from build123d import *

# Parameters (mm, degrees)
F0_R     = 1.5
F0_R_2   = 5
F1_DEPTH = 2
F2_SCALE = 10


# Not quite as in the source:
# - ends of sketch curves that miss each other by under 0.0002 mm in the source are joined


with BuildPart() as f1:
    # F0 (on Right) → F1 (new body)
    with BuildSketch(Plane.YZ):
        with BuildLine():
            Line((20.303062, 10.815357), (21.213073, 10.271883))
            ThreePointArc((21.213073, 10.271883), (21.5939035848, 10.2168943828), (21.901025054, 10.4486959684))
            Line((21.901025054, 10.4486959684), (22.426599, 11.34717))
            ThreePointArc((22.426599, 11.34717), (22.7903712384, 11.9448053837), (23.1748242578, 12.529351507))
            ThreePointArc((23.1748242578, 12.529351507), (23.8232826043, 13.8736711803), (24.046052, 15.349499))
            Line((24.046052, 15.349499), (24.046052, 15.676385))
            ThreePointArc((24.046052, 15.676385), (22.4727964344, 19.3174593718), (18.7430829675, 20.6671975356))
            ThreePointArc((18.7430829675, 20.6671975356), (15.0971647826, 20.7122553198), (11.4965779735, 21.2871678873))
            ThreePointArc((11.4965779735, 21.2871678873), (11.0304932137, 21.3939885254), (10.5631540495, 21.4951802352))
            ThreePointArc((10.5631540495, 21.4951802352), (9.7072570471, 21.5498382875), (8.8708699259, 21.360092193))
            Line((8.8708699259, 21.360092193), (6.103052, 20.297626))
            ThreePointArc((6.103052, 20.297626), (-8.8139895114, 13.1024999173), (-22.3389141406, 3.5440281676))
            Line((-22.3389141406, 3.5440281676), (-22.617202, 3.310517))
            ThreePointArc((-22.617202, 3.310517), (-23.8982246357, -0.8310495022), (-20.6544870079, -3.7071160511))
            ThreePointArc((-20.6544870079, -3.7071160511), (-17.2704039619, -4.8764379221), (-14.5151312861, -7.1628772401))
            Line((-14.5151312861, -7.1628772401), (-3.03453, -20.844925))
            ThreePointArc((-3.03453, -20.844925), (-2.3476776328, -21.3719655231), (-1.502441, -21.55935))
            Line((-1.502441, -21.55935), (2.405537, -21.55935))
            ThreePointArc((2.405537, -21.55935), (4.5268573436, -20.6806703436), (5.405537, -18.55935))
            Line((5.405537, -18.55935), (5.405537, -17.30935))
            ThreePointArc((5.405537, -17.30935), (5.3033144652, -16.5328928137), (5.0036131585, -15.8093499085))
            Line((5.0036131585, -15.8093499085), (1.781026, -10.227666))
            ThreePointArc((1.781026, -10.227666), (1.513077, -9.227666), (1.7810261443, -8.2276660833))
            Line((1.7810261443, -8.2276660833), (11.391549, 8.418247))
            ThreePointArc((11.391549, 8.418247), (13.9876851036, 10.6079458785), (17.3838640825, 10.633873234))
            ThreePointArc((17.3838640825, 10.633873234), (18.2706804185, 10.4099849641), (19.1834430004, 10.3513869851))
            ThreePointArc((19.1834430004, 10.3513869851), (19.4332447525, 10.4262916315), (19.6113513075, 10.6167898368))
            ThreePointArc((19.6113513075, 10.6167898368), (19.9150373869, 10.862970839), (20.303062, 10.815357))
        make_face()
        with Locations((2.405537, -17.30935)):
            Circle(F0_R, mode=Mode.SUBTRACT)
        with Locations((-20.58619, 0.760036)):
            Circle(F0_R, mode=Mode.SUBTRACT)
        with BuildLine():
            ThreePointArc((-0.8233559685, -5.41610236), (-8.6524240902, -3.1341370676), (-12.8829452145, 3.8375459622))
            ThreePointArc((-12.8829452145, 3.8375459622), (-11.4634165059, 5.8648445334), (-9.436118366, 4.4453149355))
            ThreePointArc((-9.436118366, 4.4453149355), (-6.5217592217, -0.3574002745), (-1.1284010077, -1.9294209114))
            ThreePointArc((-1.1284010077, -1.9294209114), (0.7674627243, -3.5202384804), (-0.8233559685, -5.41610236))
        make_face(mode=Mode.SUBTRACT)
        with Locations((-1.803858, 5.791088)):
            Circle(F0_R_2, mode=Mode.SUBTRACT)
        with Locations((19.046052, 15.349499)):
            Circle(F0_R, mode=Mode.SUBTRACT)
    extrude(amount=F1_DEPTH)


with BuildPart() as f1_1:
    # F2: moved
    add(f1.part.scale(F2_SCALE).moved(Location((0, 185.27571, -6.840324))))


solid = f1_1.part
Geometry: final body of the model. Coordinates: model frame, mm. A direction names the side the tool comes from. Round coordinates to 2 decimals unless told otherwise and drop trailing zeros. Write each loop counter-clockwise with the first axis right and the second up, starting at its lowest first coordinate (ties: lowest second). Pieces come first, ordered by that corner, then holes. Notation, with made-up numbers: M 37,37 L 75,37 A6 cw 75,42 Z; hole C 58,62 d6. An arc over 180 degrees is marked long. Write item = value, one per line.
Item 1: Access query for faces 4 (the face through (9.86, 367.86, 97.28)), 5 (the face through (10, 239.331, -186)), 6 (the face through (9.9, 99.7, -38.9)), 7 (the face through (10, 190, -222.434)), 8 (the face through (9.86, 336.76, 200.24)). Directions: +Z, -Z, +X, -X, +Y, -Y. A direction counts if a zero-diameter tool reaches every point of the face in a straight line with its end or side. Return the directions, or none.
Findings:
face_4 = -Z, +X, -X
face_5 = -Z, +X, -X, +Y
face_6 = +X, -X
face_7 = -Z, +X, -X, +Y, -Y
face_8 = +Z, +X, -X
Item 2: Material intervals for line 1 along Y through (x, z) = (3.75, 0); line 2 along Z through (x, y) = (11, 211); line 3 along Z through (x, y) = (7.25, 133.5), sorted ascending. Write a range as [from, to].
Findings:
line_1 = [-54.94, -35.57], [-5.61, 67], [108.94, 254.54]
line_2 = [-222.39, -194.84], [-165.03, -122.82], [-75.41, 26.89], [75.25, 181.81]
line_3 = [-189.75, -56.25], [-18.7, 14.17], [87.97, 144.6]
Item 3: Section query A-A on y = 110. Return loops of the section in (x, z), then the cut area to 3 significant figures.
Findings:
outline = M 0,-161.74 L 20,-161.74 L 20,-45.78 L 0,-45.78 Z; M 0,-1.18 L 20,-1.18 L 20,131.63 L 0,131.63 Z
area = 4,980 mm^2
Item 4: Pin query (flat end, axial travel): P1, Ø5, axis at x = 8, y = 138, coming from the +Z side; P2, Ø1, axis at x = 3.5, y = 136.5, coming from the +Z side; P3, Ø8, axis at x = 12, y = 154, coming from the +Z side; P4, Ø24, axis at y = -20.59, z = 0.76, coming from the +X side. Return the tip coordinate at first contact, or that it passes through.
Findings:
P1 = 148.3
P2 = 146.46
P3 = 157.25
P4 = through
Item 5: Section query C-C on x = 8.25. State how many separate pieces and enclosed holes the cut face has, then the cut area to 3 significant figures.
Findings:
separate_pieces = 1
enclosed_holes = 5
area = 77,800 mm^2
Item 6: Section query D-D on z = -133. Return loops of the section in (x, y).
Findings:
outline = M 0,85.88 L 20,85.88 L 20,216.87 L 0,216.87 Z
Item 7: Pull-direction query (Y, two-part tool) for faces 1 (the face through (9.86, 223.187, -185.679)), 2 (the face through (9.86, 99.14, 125.36)), 3 (the face through (0, 166, -6)); classes: pulls with the +Y half, pulls with the -Y half, needs draft (parallel to the pull), parting line crosses it, or undercut.
Findings:
face_1 = undercut
face_2 = pulls with the -Y half
face_3 = needs draft
Item 8: Section query B-B on z = 57.5. Return loops of the section in (x, y), then the cut area to 3 significant figures.
Findings:
outline = M 0,-2.01 L 20,-2.01 L 20,117.65 L 0,117.65 Z; M 0,216.82 L 20,216.82 L 20,287.74 L 0,287.74 Z
area = 3,810 mm^2
